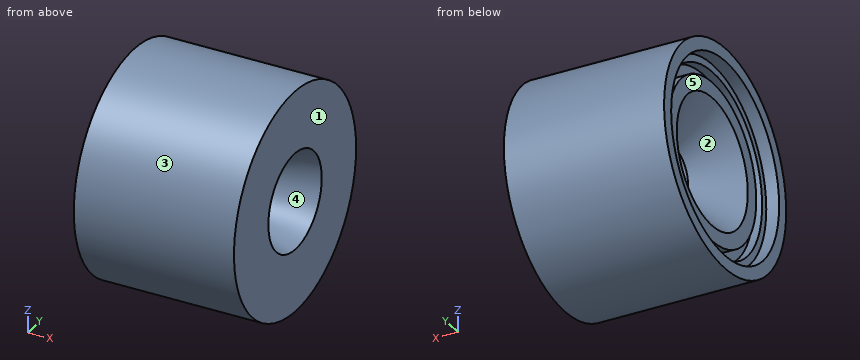
```python
from build123d import *

# Parameters (mm, degrees)
SKETCH2_R          = 22.2885
SKETCH2_R_2        = 19.6723
CUT_EXTRUDE1_DEPTH = 2.286


with BuildPart() as part:
    # Sketch1 → Revolve1 (revolve)
    with BuildSketch(Plane.XY):
        Polygon((0, 24.13), (3.175, 24.13), (3.175, 15.875), (12.7, 6.35), (18.796, 6.35), (39.650699913, 11.938), (39.650699913, 27.305), (0, 27.305), align=None)
    revolve(axis=Axis((0, 0, 0), (1, 0, 0)))

    # Sketch2 → Cut-Extrude1 (cut)
    with BuildSketch(Plane.ZY.offset(-3.175)):
        Circle(SKETCH2_R)
        Circle(SKETCH2_R_2, mode=Mode.SUBTRACT)
    extrude(amount=-CUT_EXTRUDE1_DEPTH, mode=Mode.SUBTRACT)


solid = part.part
```
The model under review builds one solid part; all positions refer to its coordinate system, in mm. Face numbers are marked on the shaded views. A direction names the side the tool comes from. Round coordinates to 2 decimals unless told otherwise and drop trailing zeros. Write each loop counter-clockwise with the first axis right and the second up, starting at its lowest first coordinate (ties: lowest second). Pieces come first, ordered by that corner, then holes.
(1) We need section D-D on y = 23. Give the boundary of the cut face in (x, z) (3 decimals).
(2) Wall thickness on L1, parallel to Z at x = 17, y = 0 (3 decimals); L2, parallel to Z at x = 1, y = 0 (3 decimals); L3, parallel to X at y = 15.5, z = 8.5 (3 decimals): over which ranges is each line inside the solid? List them lowest first.
(3) Mouldability with a two-part tool opening along Y and no side actions: class the marked faces 1, 2 and 3 as +Y half, -Y half, draft (parallel to the pull), parting line (faces both ways), or undercut.
(4) Machinability: for the marked faces 4 and 5, which of the approach directions +Z, -Z, +X, -X, +Y, -Y give a long, thin tool a straight path to every point of the face, cutting with its end or side? Answer none if there is none.
(5) Insertion check: pin 1 (2 mm diameter, centred on x = 16.5, y = 21.5, fed in from -Z); pin 2 (6 mm diameter, centred on x = 18.5, y = -13.5, fed in from -Z); pin 3 (4 mm diameter, centred on x = 28.5, y = -12.5, fed in from +Z); pin 4 (7.5 mm diameter, centred on y = 0, z = 0, fed in from -X). Each pin has a flat end and moves straight along its axis. Give the tip position at first contact, or say it passes through.
(6) We need section C-C on x = 4.5. Give the number of separate pieces and of enclosed holes in the cut face, and give its area (3 significant figures).
Findings below:
1. outline: (0, -14.716) - (39.651, -14.716) - (39.651, 14.716) - (0, 14.716) - (0, 7.298) - (3.175, 7.298) - (3.175, -7.298) - (0, -7.298) - close
2. L1: z = -27.305 to -6.35, 6.35 to 27.305
2. L2: z = -27.305 to -24.13, 24.13 to 27.305
2. L3: x = 3.175 to 39.651
3. face 1: draft
3. face 2: undercut
3. face 3: parting line
4. face 4: +X
4. face 5: -X
5. pin 1: stops at z = -18.04
5. pin 2: stops at z = -25.21
5. pin 3: stops at z = 25.21
5. pin 4: passes through
6. separate pieces: 2
6. enclosed holes: 2
6. area: 1,330 mm2
